from build123d import *

# Parameters (mm, degrees)
SZKIC3_W                   = 2
SZKIC3_H                   = 10
SZKIC5_R                   = 1.4
WYTNIJ_WYCI_GNI_CIE1_DEPTH = 100
ZAOKR_GLENIE1_R            = 0.5


with BuildPart() as part:
    # Wyciągnięcie po ścieżce1: sweep along a path in Szkic2
    with BuildLine(Plane(origin=(0, 0, 0), x_dir=(1, 0, 0), z_dir=(0, 1, 0))) as wyci_gni_cie_po_cie_ce1_path:
        Line((0, 0), (0, 25))
        ThreePointArc((0, 25), (35, 60), (70, 25))
        Line((70, 25), (70, 0))
    # Szkic3 → Wyciągnięcie po ścieżce1 (sweep)
    with BuildSketch(Plane.XY):
        Rectangle(SZKIC3_W, SZKIC3_H)
    sweep(path=wyci_gni_cie_po_cie_ce1_path.line)

    # Szkic5 → Wytnij-wyciągnięcie1 (cut)
    with BuildSketch(Plane.ZY.offset(1)):
        with Locations(Location((-5, 0, 0), (0, 0, 270))):
            Circle(SZKIC5_R)
    extrude(amount=-WYTNIJ_WYCI_GNI_CIE1_DEPTH, mode=Mode.SUBTRACT)

    # Zaokrąglenie1
    zaokr_glenie1_edges = [part.edges().sort_by_distance(p)[0] for p in [
        (35, -5, -61),
        (35, 5, -61),
        (1, 0, 0),
        (-1, 0, 0),
        (0, -5, 0),
        (1, -5, -12.5),
        (35, -5, -59),
        (70, -5, 0),
        (71, -5, -12.5),
        (71, 0, 0),
        (71, 5, -12.5),
        (70, 5, 0),
        (69, 0, 0),
        (69, -5, -12.5),
        (69, 5, -12.5),
        (-1, -5, -12.5),
        (35, 5, -59),
        (1, 5, -12.5),
        (-1, 5, -12.5),
    ]]
    fillet(zaokr_glenie1_edges, radius=ZAOKR_GLENIE1_R)


solid = part.part
Input: part model. Units: mm. Frame: model coordinates. A direction names the side the tool comes from. Coordinates: 2 decimals unless noted, no trailing zeros. Order: outer loops, then holes, each group sorted by start corner. A loop starts at its lowest first (then second) coordinate and runs counter-clockwise, first axis right, second up. Notation, with made-up numbers: M 54.25,26 L 86.25,26 A17 cw 86.25,55 Z; hole C -16.5,2.5 d2. An arc over 180 degrees is marked long. Answer in a Markdown table with one row per item.
(1) Section query B-B, the plane y = 0. Output: boundary loops of the cut face in (x, z), plus the area to 3 significant figures.
Numbers:
| item | result |
|---|---|
| outline | M -1,-25 A36 ccw 71,-25 L 71,-6.4 L 69,-6.4 L 69,-25 A34 cw 1,-25 L 1,-6.4 L -1,-6.4 Z; M -1,-3.6 L 1,-3.6 L 1,-0.5 A0.5 ccw 0.5,0 L -0.5,0 A0.5 ccw -1,-0.5 Z; M 69,-3.6 L 71,-3.6 L 71,-0.5 A0.5 ccw 70.5,0 L 69.5,0 A0.5 ccw 69,-0.5 Z |
| area | 308 mm^2 |
(2) Material intervals for line 1 (X direction, y = 2, z = -4.5); line 2 (Z direction, x = 35, y = 3.75); line 3 (X direction, y = -0.25, z = -46), sorted ascending. Write a range as [from, to].
Numbers:
| item | result |
|---|---|
| line 1 | x = [-1, 1], [69, 71] |
| line 2 | z = [-61, -59] |
| line 3 | x = [5.76, 8.26], [61.74, 64.24] |
(3) Section query C-C, the plane z = -5. Output: boundary loops of the cut face in (x, y).
Numbers:
| item | result |
|---|---|
| outline | M -1,-4.5 A0.5 ccw -0.5,-5 L 0.5,-5 A0.5 ccw 1,-4.5 L 1,-1.4 L -1,-1.4 Z; M -1,1.4 L 1,1.4 L 1,4.5 A0.5 ccw 0.5,5 L -0.5,5 A0.5 ccw -1,4.5 Z; M 69,-4.5 A0.5 ccw 69.5,-5 L 70.5,-5 A0.5 ccw 71,-4.5 L 71,-1.4 L 69,-1.4 Z; M 69,1.4 L 71,1.4 L 71,4.5 A0.5 ccw 70.5,5 L 69.5,5 A0.5 ccw 69,4.5 Z |
(4) Section query A-A, the plane z = -19. Output: boundary loops of the cut face in (x, y).
Numbers:
| item | result |
|---|---|
| outline | M -1,-4.5 A0.5 ccw -0.5,-5 L 0.5,-5 A0.5 ccw 1,-4.5 L 1,4.5 A0.5 ccw 0.5,5 L -0.5,5 A0.5 ccw -1,4.5 Z; M 69,-4.5 A0.5 ccw 69.5,-5 L 70.5,-5 A0.5 ccw 71,-4.5 L 71,4.5 A0.5 ccw 70.5,5 L 69.5,5 A0.5 ccw 69,4.5 Z |
(5) Section query D-D, the plane x = 35. Output: boundary loops of the cut face in (y, z), plus the area to 3 significant figures.
Numbers:
| item | result |
|---|---|
| outline | M -5,-60.5 A0.5 ccw -4.5,-61 L 4.5,-61 A0.5 ccw 5,-60.5 L 5,-59.5 A0.5 ccw 4.5,-59 L -4.5,-59 A0.5 ccw -5,-59.5 Z |
| area | 19.8 mm^2 |
(6) Access query for faces 4 (the cylindrical face through (69.986, 0.303, -6.367)), 5 (the flat face through (69, 0, -13)). Directions: +Z, -Z, +X, -X, +Y, -Y. A direction counts if a zero-diameter tool reaches every point of the face in a straight line with its end or side. Return the directions, or none.
Numbers:
| item | result |
|---|---|
| face 4 | +X, -X |
| face 5 | +Z, +Y, -Y |
(7) Contact query for flat-ended pins moving along their axis: pin 1 Ø2 at (y, z) = (0, -28.5) entering from +X; pin 2 Ø1.5 at (y, z) = (-3, -30.5) entering from +X; pin 3 Ø1.5 at (x, y) = (14, 2) entering from +Z; pin 4 Ø1.7 at (y, z) = (0, -5) entering from +X. Output: stop coordinate, or through.
Numbers:
| item | result |
|---|---|
| pin 1 | stops at x = 70.91 |
| pin 2 | stops at x = 70.69 |
| pin 3 | stops at z = -51.13 |
| pin 4 | passes through |
(8) Draft query along X for faces 1 (the flat face through (1, 0, -13)), 2 (the flat face through (32, -5, -60)), 3 (the cylindrical face through (34.21, -0.06, -60.99)). Return one class per face: pulls with the +X half, pulls with the -X half, needs draft (parallel to the pull), parting line crosses it, or undercut.
Numbers:
| item | result |
|---|---|
| face 1 | undercut |
| face 2 | needs draft |
| face 3 | parting line crosses it |
